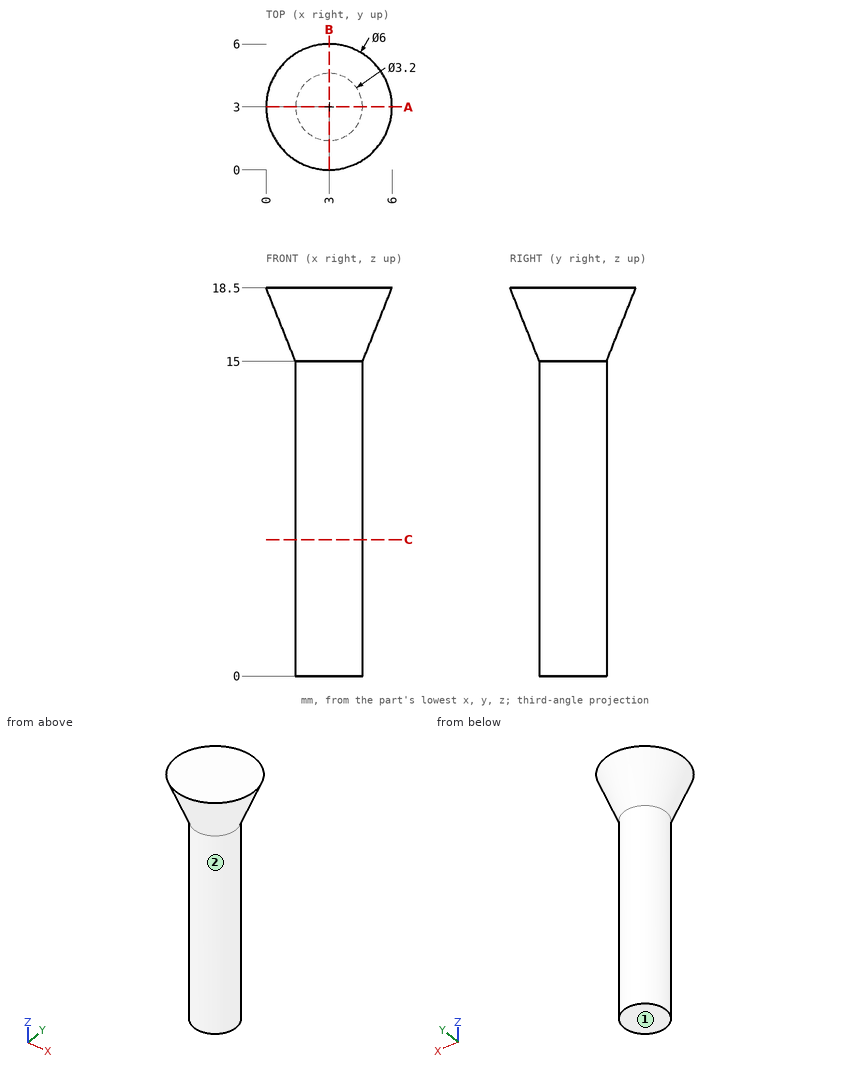
The figure shows three views and two pictorial views of one solid part (mm, origin at its lowest corner). Answer the questions. Give positions to 0.01 mm unless a question says otherwise; leave off trailing zeros. Loops run counter-clockwise (first coordinate to the right, second up) from the corner with the lowest first, then second, coordinate; pieces in that order, holes last. Notation, with made-up numbers: (59.5, 53.5) - (94.5, 53.5) arc R21 cw to (94.5, 81.5) - close; hole circle Ø2 at (-33.5, -17.75). An arc over 180 degrees is marked (long way). Use one line per item in the form item = value.
1. Section C-C on z = 6.5 is taken. Give the vertices of the cut face in (x, y).
Calculated:
outline = circle Ø3.2 at (3, 3)
2. Find the intervals of material crossed by line 1 along Z through (x, y) = (4.35, 5.3); line 2 along Z through (x, y) = (5.35, 2.4); line 3 along X through (y, z) = (1.6, 7.25), in increasing order. Write a range as [from, to].
Calculated:
line_1 = [17.67, 18.5]
line_2 = [17.06, 18.5]
line_3 = [2.23, 3.77]
3. The mould has two halves that part along Y. Classify the marked faces 1 and 2: pulls with the +Y half, pulls with the -Y half, needs draft (parallel to the pull), parting line crosses it, or undercut.
Calculated:
face_1 = needs draft
face_2 = parting line crosses it
4. Section A-A on y = 3 is taken. Give the vertices of the cut face in (x, z), then the cut area to 3 significant figures.
Calculated:
outline = (0, 18.5) - (1.4, 15) - (1.4, 0) - (4.6, 0) - (4.6, 15) - (6, 18.5) - close
area = 64.1 mm^2
5. Given pin 1 Ø2 at (y, z) = (5, 16) entering from +X, flat-ended and moving along its own axis, determine where the tip first touches the part or whether it passes through.
Calculated:
pin_1 = 4.89
